Verification items for the finished model (mm, model axes). A direction names the side the tool comes from. Give positions to 0.01 mm unless a question says otherwise; leave off trailing zeros. Order: outer loops, then holes, each group sorted by start corner. A loop starts at its lowest first (then second) coordinate and runs counter-clockwise, first axis right, second up.
(1) Access from +Z, -Z, +X, -X, +Y, -Y to the whole of each face (thin tool, end or side, straight path). Record for faces 1 (the face through (9.586, -3.718, -3.019)), 2 (the face through (11, 4, 10)), 3 (the face through (-2, -6, -5)), 4 (the face through (-1.25, 0, -6)).
(2) Mould release check, pull along Z, two halves, no side actions. Record for faces 5 (the face through (-9, 0, 9)), 6 (the face through (-4.78, 2.434, 21.526)), 7 (the face through (-2.018, 5.907, -15.368)): pulls with the +Z half, pulls with the -Z half, needs draft (parallel to the pull), parting line crosses it, or undercut.
(3) Sectioned sample at B-B on z = 0. Record the cut outline in (x, y).
(4) Scan lines: L1, parallel to Z at x = 0, y = -3; L2, parallel to Z at x = -6, y = 3.5 (3 decimals); L3, parallel to X at y = 4, z = -3. Record each from-to range of solid material in increasing order.
(5) Gauge pin test, flat ends, axial feed: pin 1 (6 mm diameter, centred on x = -8.15, z = 8.15, fed in from +Y); pin 2 (2 mm diameter, centred on x = 2, z = 14, fed in from -Y); pin 3 (0.5 mm diameter, centred on y = 0, z = -5.5, fed in from +X). Record the tip position at first contact, or that the pin passes through.
(6) Sectioned sample at C-C on y = 2.25. Record the cut outline in (x, z), plus the area to 3 significant figures.
(7) Sectioned sample at A-A on x = 0. Record the cut outline in (y, z), plus the area to 3 significant figures.
```python
from build123d import *

# Parameters (mm, degrees)
FILLET1_R               = 1.5
SKETCH2_W               = 2.5
SKETCH2_H               = 1.5
CUT_EXTRUDE1_DEPTH      = 7.84
CUT_EXTRUDE1_DEPTH_BACK = 7
SKETCH3_R               = 3.4
CUT_EXTRUDE2_DEPTH      = 2.2
CIRPATTERN1_COUNT       = 4


with BuildPart() as part:
    # Sketch1 → Revolve1 (revolve)
    with BuildSketch(Plane.XY):
        Polygon((5, -6), (10.05, -6), (10.05, 0), (22.05, 0), (22.05, 4.8), (15.5, 6.84), (15.5, 5), (5, 5), align=None)
    revolve(axis=Axis((0, 0, 0), (0, 1, 0)))

    # Fillet1
    fillet1_edges = [part.edges().sort_by_distance(p)[0] for p in [
        (-10.05, 0, 0),
    ]]
    fillet(fillet1_edges, radius=FILLET1_R)

    # Sketch2 → Cut-Extrude1 (cut, two sides)
    with BuildSketch(Plane(origin=(0, 0, 0), x_dir=(1, 0, 0), z_dir=(0, 1, 0))) as cut_extrude1_sk:
        with Locations((0, 5.591229183)):
            Rectangle(SKETCH2_W, SKETCH2_H)
    extrude(amount=CUT_EXTRUDE1_DEPTH, mode=Mode.SUBTRACT)
    extrude(cut_extrude1_sk.sketch, amount=-CUT_EXTRUDE1_DEPTH_BACK, mode=Mode.SUBTRACT)

    # Sketch3 → Cut-Extrude2 (cut)
    with BuildSketch(Plane(origin=(0, 5, 0), x_dir=(1, 0, 0), z_dir=(0, 1, 0))):
        with Locations((8.149405653, 8.149405653)):
            Circle(SKETCH3_R)
    cut_extrude2 = extrude(amount=-CUT_EXTRUDE2_DEPTH, mode=Mode.SUBTRACT)

    # CirPattern1: Cut-Extrude2 ×4 about axis
    cirpattern1_axis = Axis((0, 0, 0), (0, 1, 0))
    for i in range(1, CIRPATTERN1_COUNT):
        add(cut_extrude2.rotate(cirpattern1_axis, i * 360 / CIRPATTERN1_COUNT), mode=Mode.SUBTRACT)


solid = part.part
```
Ans:
1. face 1: -Y
1. face 2: +Y
1. face 3: +Z, -Z, +X, -X, -Y
1. face 4: +Y, -Y
2. face 5: needs draft
2. face 6: parting line crosses it
2. face 7: undercut
3. outline: (-22.05, 0) - (-11.55, 0) arc R1.5 cw to (-10.05, -1.5) - (-10.05, -6) - (-5, -6) - (-5, 5) - (-15.5, 5) - (-15.5, 6.84) - (-22.05, 4.8) - close; (5, -6) - (10.05, -6) - (10.05, -1.5) arc R1.5 cw to (11.55, 0) - (22.05, 0) - (22.05, 4.8) - (15.5, 6.84) - (15.5, 5) - (5, 5) - close
4. L1: z = -10.05 to -6.34, 5 to 10.05
4. L2: z = -21.218 to -10.784, -5.515 to 5.515, 10.784 to 21.218
4. L3: x = -21.84 to -4, 4 to 21.84
5. pin 1: stops at y = 2.8
5. pin 2: stops at y = 0
5. pin 3: stops at x = 21.42
6. outline: circle Ø44.1 at (0, 0); hole (-1.25, -6.34) - (1.25, -6.34) - (1.25, -4.84) arc R5 ccw (long way) to (-1.25, -4.84) - close
6. area: 1,450 mm2
7. outline: (-6, -10.05) - (-1.5, -10.05) arc R1.5 cw to (0, -11.55) - (0, -22.05) - (4.8, -22.05) - (6.84, -15.5) - (5, -15.5) - (5, -6.34) - (-6, -6.34) - close; (-6, 5) - (5, 5) - (5, 15.5) - (6.84, 15.5) - (4.8, 22.05) - (0, 22.05) - (0, 11.55) arc R1.5 cw to (-1.5, 10.05) - (-6, 10.05) - close
7. area: 228 mm2
